Here's how the part is built. I have some questions about the finished solid (model axes, mm). Face numbers are marked on the shaded views. A direction names the side the tool comes from. Round coordinates to 2 decimals unless told otherwise and drop trailing zeros. Order: outer loops, then holes, each group sorted by start corner. A loop starts at its lowest first (then second) coordinate and runs counter-clockwise, first axis right, second up. Notation, with made-up numbers: (-34.75, 65.5) -> (-7.75, 65.5) arc R20 ccw to (-7.75, 76.5) -> close; hole circle Ø8 at (30, 47.5). An arc over 180 degrees is marked (long way). One line per item, written item: value.
```python
from build123d import *

# Parameters (mm, degrees)
SKETCH1_R                   = 21.25
SKETCH1_R_2                 = 19.25
BOSS_EXTRUDE1_DEPTH         = 3.25
SKETCH4_R                   = 7
CUT_EXTRUDE2_DEPTH          = 8
SKETCH5_R                   = 7
CUT_EXTRUDE3_DEPTH          = 2
SKETCH7_R                   = 8.5
BOSS_EXTRUDE2_DEPTH         = 16
SKETCH6_R                   = 6.6675
CUT_EXTRUDE5_DEPTH          = 36.540444334
F_33_0_113_DIAMETER_HOLE1_D = 2.8702


with BuildPart() as part:
    # Sketch1 → Boss-Extrude1 (new body)
    with BuildSketch(Plane.XY):
        with Locations(Location((0, 0, 0), (0, 0, 180))):
            Circle(SKETCH1_R)
        with Locations(Location((0, 0, 0), (0, 0, 180))):
            Circle(SKETCH1_R_2, mode=Mode.SUBTRACT)
    extrude(amount=BOSS_EXTRUDE1_DEPTH)

    # Sketch2 → Revolve1 (revolve)
    with BuildSketch(Plane(origin=(0, 0, 0), x_dir=(1, 0, 0), z_dir=(0, 1, 0))):
        Polygon((-21.25, 0), (-15.7, 9.5), (0, 9.5), (0, 6.526382134), (-15.7, 6.526382134), (-19.512781141, 0), align=None)
    revolve(axis=Axis((0, 0, -9.5), (0, 0, 1)))

    # Sketch4 → Cut-Extrude2 (cut)
    with BuildSketch(Plane(origin=(0, 0, -9.5), x_dir=(-1, 0, 0), z_dir=(0, 0, -1))):
        with Locations((0, 16.5)):
            Circle(SKETCH4_R)
        with Locations((16.5, 0)):
            Circle(SKETCH4_R)
        with Locations((0, -16.5)):
            Circle(SKETCH4_R)
    extrude(amount=-CUT_EXTRUDE2_DEPTH, mode=Mode.SUBTRACT)

    # Sketch5 → Cut-Extrude3 (cut)
    with BuildSketch(Plane(origin=(0, 0, -9.5), x_dir=(-1, 0, 0), z_dir=(0, 0, -1))):
        with Locations((-16.5, 0)):
            Circle(SKETCH5_R)
    extrude(amount=-CUT_EXTRUDE3_DEPTH, mode=Mode.SUBTRACT)

    # Sketch7 → Boss-Extrude2 (add)
    with BuildSketch(Plane.XY.offset(-6.526382134)):
        Circle(SKETCH7_R)
    extrude(amount=BOSS_EXTRUDE2_DEPTH)

    # Sketch6 → Cut-Extrude5 (cut, through all)
    with BuildSketch(Plane(origin=(0, 0, -9.5), x_dir=(-1, 0, 0), z_dir=(0, 0, -1))):
        Circle(SKETCH6_R)
    extrude(amount=-CUT_EXTRUDE5_DEPTH, mode=Mode.SUBTRACT)

    # #33 (0.113) Diameter Hole1 (through all)
    with Locations(Plane(origin=(0, 0, -9.5), x_dir=(-1, 0, 0), z_dir=(0, 0, -1))):
        with Locations((7.778174593, 7.778174593), (7.778174593, -7.778174593), (-7.778174593, -7.778174593), (-7.778174593, 7.778174593)):
            Hole(F_33_0_113_DIAMETER_HOLE1_D / 2)


solid = part.part
```
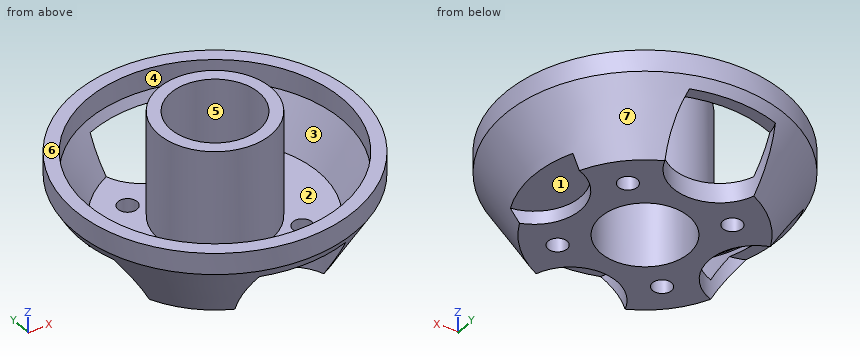
Q1. I want a section at C-C on x = 0. Write out the boundary of the cut face in (y, z), then the cut area to 3 significant figures.
Answers:
outline: (-21.25, 0) -> (-20.37, -1.5) -> (-18.64, -1.5) -> (-19.51, 0) -> (-19.25, 0) -> (-19.25, 3.25) -> (-21.25, 3.25) -> close; (-9.5, -9.5) -> (-6.67, -9.5) -> (-6.67, 9.47) -> (-8.5, 9.47) -> (-8.5, -6.53) -> (-9.5, -6.53) -> close; (6.67, -9.5) -> (9.5, -9.5) -> (9.5, -6.53) -> (8.5, -6.53) -> (8.5, 9.47) -> (6.67, 9.47) -> close; (18.64, -1.5) -> (20.37, -1.5) -> (21.25, 0) -> (21.25, 3.25) -> (19.25, 3.25) -> (19.25, 0) -> (19.51, 0) -> close
area: 93.7 mm2
Q2. For P1, Ø6, axis at x = -3.5, y = 14, coming from the +Z side; P2, Ø1, axis at x = -2, z = -0.5, coming from the -Y side; P3, Ø5, axis at x = 8.5, z = -5.5, coming from the +Y side; P4, Ø10.5, axis at x = 0, y = 0, coming from the +Z side, each with a flat end and sliding along its axis, tell me the tip position at first contact or that it passes through.
Answers:
P1: z = -6.53
P2: y = -21.16
P3: y = 17.89
P4: through
Q3. I want a section at D-D on y = 5.5. Give the number of separate pieces and of enclosed holes in the cut face, then the cut area to 3 significant figures.
Answers:
separate pieces: 3
enclosed holes: 0
area: 169 mm2
Q4. If we mould it in two halves opening along X, with no side actions, what happens to the marked faces 4, 5, 6 and 7? For each: pulls with the +X half, pulls with the -X half, needs draft (parallel to the pull), parting line crosses it, or undercut.
Answers:
face 4: undercut
face 5: undercut
face 6: needs draft
face 7: parting line crosses it
Q5. I want a section at B-B on y = 0. Write out the boundary of the cut face in (x, z).
Answers:
outline: (-21.25, 0) -> (-20.37, -1.5) -> (-18.64, -1.5) -> (-19.51, 0) -> (-19.25, 0) -> (-19.25, 3.25) -> (-21.25, 3.25) -> close; (-9.5, -9.5) -> (-6.67, -9.5) -> (-6.67, 9.47) -> (-8.5, 9.47) -> (-8.5, -6.53) -> (-9.5, -6.53) -> close; (6.67, -9.5) -> (9.5, -9.5) -> (9.5, -7.5) -> (16.87, -7.5) -> (21.25, 0) -> (21.25, 3.25) -> (19.25, 3.25) -> (19.25, 0) -> (19.51, 0) -> (15.7, -6.53) -> (8.5, -6.53) -> (8.5, 9.47) -> (6.67, 9.47) -> close
Q6. Which directions (+Z, -Z, +X, -X, +Y, -Y) give clear straight access to the entire face, cutting with the end or side of a thin tool? Please do the marked faces 1, 2 and 3.
Answers:
face 1: -Z, +X
face 2: +Z
face 3: none
Q7. I want a section at A-A on z = -3. Write out the boundary of the cut face in (x, y) (1 decimal).
Answers:
outline: (-18.3, -6.8) arc R19.5 ccw to (-6.8, -18.3) arc R7 cw to (-7, -16.3) arc R17.8 cw to (-16.3, -7) arc R7 cw to start; (-18.3, 6.8) arc R7 cw to (-16.3, 7) arc R17.8 cw to (-7, 16.3) arc R7 cw to (-6.8, 18.3) arc R19.5 ccw to start; circle Ø17 at (0, 0); (6.8, -18.3) arc R19.5 ccw to (6.8, 18.3) arc R7 cw to (7, 16.3) arc R17.8 cw to (7, -16.3) arc R7 cw to start; hole circle Ø13.3 at (0, 0)
Q8. I need wall thicknesses on line 1 along Y through (x, z) = (0, 2.15); line 2 along Y through (x, z) = (0, -6.25); line 3 along X through (y, z) = (4.5, 2). Which ranges of each line are inside material? Lowest first, please.
Answers:
line 1: -21.25 to -19.25, -8.5 to -6.67, 6.67 to 8.5, 19.25 to 21.25
line 2: -8.5 to -6.67, 6.67 to 8.5
line 3: -20.77 to -18.72, -7.21 to -4.92, 4.92 to 7.21, 18.72 to 20.77
